Can you work these out from the model? Positions are in its coordinate system, mm. Face numbers are marked on the shaded views. Give positions to 0.01 mm unless a question says otherwise; leave off trailing zeros. Loops run counter-clockwise (first coordinate to the right, second up) from the corner with the lowest first, then second, coordinate; pieces in that order, holes last. Notation, with made-up numbers: (-31.5, 28.25) -> (24.5, 28.25) arc R21 ccw to (24.5, 59.25) -> close; hole circle Ø9 at (-12.5, 55.25). An arc over 180 degrees is marked (long way). Use CSV: the item, a comma, the result in double quotes.
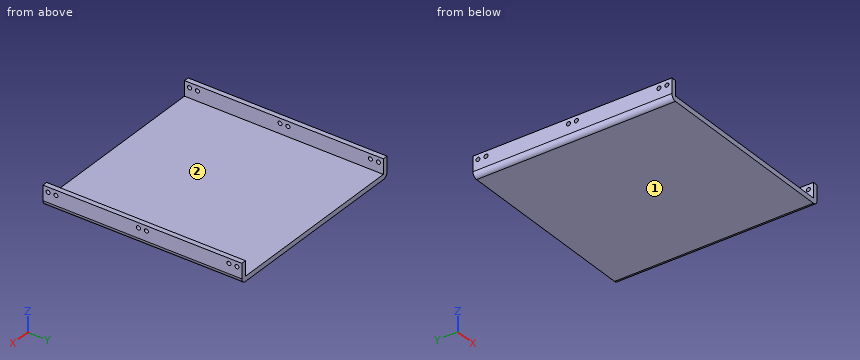
from build123d import *

# Parameters (mm, degrees)
BOSS_EXTRUDE1_DEPTH = 100
SKETCH4_R           = 2
CUT_EXTRUDE1_DEPTH  = 214


with BuildPart() as part:
    # Sketch3 → Boss-Extrude1 (new, symmetric)
    with BuildSketch(Plane(origin=(0, 0, 0), x_dir=(1, 0, 0), z_dir=(0, 1, 0))):
        with BuildLine():
            Line((95, 0), (-95, 0))
            ThreePointArc((-95, 0), (-98.535533906, -1.464466094), (-100, -5))
            Line((-100, -5), (-100, -20))
            Line((-100, -20), (-95, -20))
            Line((-95, -20), (-95, -5))
            Line((-95, -5), (95, -5))
            Line((95, -5), (95, -20))
            Line((95, -20), (100, -20))
            Line((100, -20), (100, -5))
            ThreePointArc((100, -5), (98.535533906, -1.464466094), (95, 0))
        make_face()
    extrude(amount=BOSS_EXTRUDE1_DEPTH, both=True)

    # Sketch4 → Cut-Extrude1 (cut)
    with BuildSketch(Plane.ZY.offset(100)):
        with Locations((15, 95)):
            Circle(SKETCH4_R)
        with Locations((15, 87)):
            Circle(SKETCH4_R)
        with Locations((15, 4)):
            Circle(SKETCH4_R)
        with Locations((15, -4)):
            Circle(SKETCH4_R)
        with Locations((15, -95)):
            Circle(SKETCH4_R)
        with Locations((15, -87)):
            Circle(SKETCH4_R)
    extrude(amount=-CUT_EXTRUDE1_DEPTH, mode=Mode.SUBTRACT)


solid = part.part
(1) Will these pins go through, and if not, where does the flat tip stop? pin 1 Ø2.5 at (y, z) = (87, 15) entering from +X; pin 2 Ø1 at (x, y) = (62, -62.5) entering from +Z; pin 3 Ø1.5 at (y, z) = (-45.5, 2.5) entering from -X.
Answer sheet:
pin 1,"passes through"
pin 2,"stops at z = 5"
pin 3,"stops at x = -99.68"
(2) If I drill on L1, parallel to X at y = -2.5, z = 10; L2, parallel to Z at x = 60.5, y = 81; L3, parallel to X at y = 90.5, z = 3, over which ranges is the centre line in solid material (lowest first)? Write a range as from..to.
Answer sheet:
L1,"x = -100..-95, 95..100"
L2,"z = 0..5"
L3,"x = -99.58..99.58"
(3) If we section it at B-B, the plane y = -12: Write out the boundary of the cut face in (x, z).
Answer sheet:
outline,"(-100, 5) arc R5 ccw to (-95, 0) -> (95, 0) arc R5 ccw to (100, 5) -> (100, 20) -> (95, 20) -> (95, 5) -> (-95, 5) -> (-95, 20) -> (-100, 20) -> close"
(4) If we section it at A-A, the plane z = 8: Write out the boundary of the cut face in (x, y).
Answer sheet:
outline,"(-100, -100) -> (-95, -100) -> (-95, 100) -> (-100, 100) -> close; (95, -100) -> (100, -100) -> (100, 100) -> (95, 100) -> close"
(5) If we section it at C-C, the plane x = 45: Write out the boundary of the cut face in (y, z).
Answer sheet:
outline,"(-100, 0) -> (100, 0) -> (100, 5) -> (-100, 5) -> close"
(6) We'd pull the mould along X, two halves only. Please class the marked faces 1 and 2: released by +X, released by -X, zero draft, split by the parting line, or undercut.
Answer sheet:
face 1,"zero draft"
face 2,"undercut"
